Source: three-view drawing plus pictorial views. Frame: mm from the lowest corner of the part. A direction names the side the tool comes from. Give positions to 0.01 mm unless a question says otherwise; leave off trailing zeros. Order: outer loops, then holes, each group sorted by start corner. A loop starts at its lowest first (then second) coordinate and runs counter-clockwise, first axis right, second up. Notation, with made-up numbers: (7.5, 87.25) - (66.5, 87.25) arc R10 ccw to (66.5, 104.25) - close; hole circle Ø6 at (-17.75, -6.75). An arc over 180 degrees is marked (long way). Answer in a Markdown table with one row per item. Add a question column.
1. Contact query for flat-ended pins moving along their axis: pin 1 (4 mm diameter, centred on y = 3, z = 19.5, fed in from -X); pin 2 (3 mm diameter, centred on y = 7, z = 5, fed in from -X); pin 3 (2 mm diameter, centred on x = 11, z = 12, fed in from -Y). Output: stop coordinate, or through.
2. Section query A-A on x = 6.35. Return loops of the section in (y, z), and give its area (3 significant figures).
3. Access query for the marked faces 1 and 2. Directions: +Z, -Z, +X, -X, +Y, -Y. A direction counts if a zero-diameter tool reaches every point of the face in a straight line with its end or side. Return the directions, or none.
4. Ray query, line 1 (Z direction, x = 3, y = 2.75); line 2 (X direction, y = 10, z = 20.25); line 3 (X direction, y = 4, z = 12.75). Return the intervals inside material, ascending. Write a range as [from, to].
5. Section query C-C on z = 5.5. Return loops of the section in (x, y), and give its area (3 significant figures).
6. Section query D-D on y = 1. Return loops of the section in (x, z).
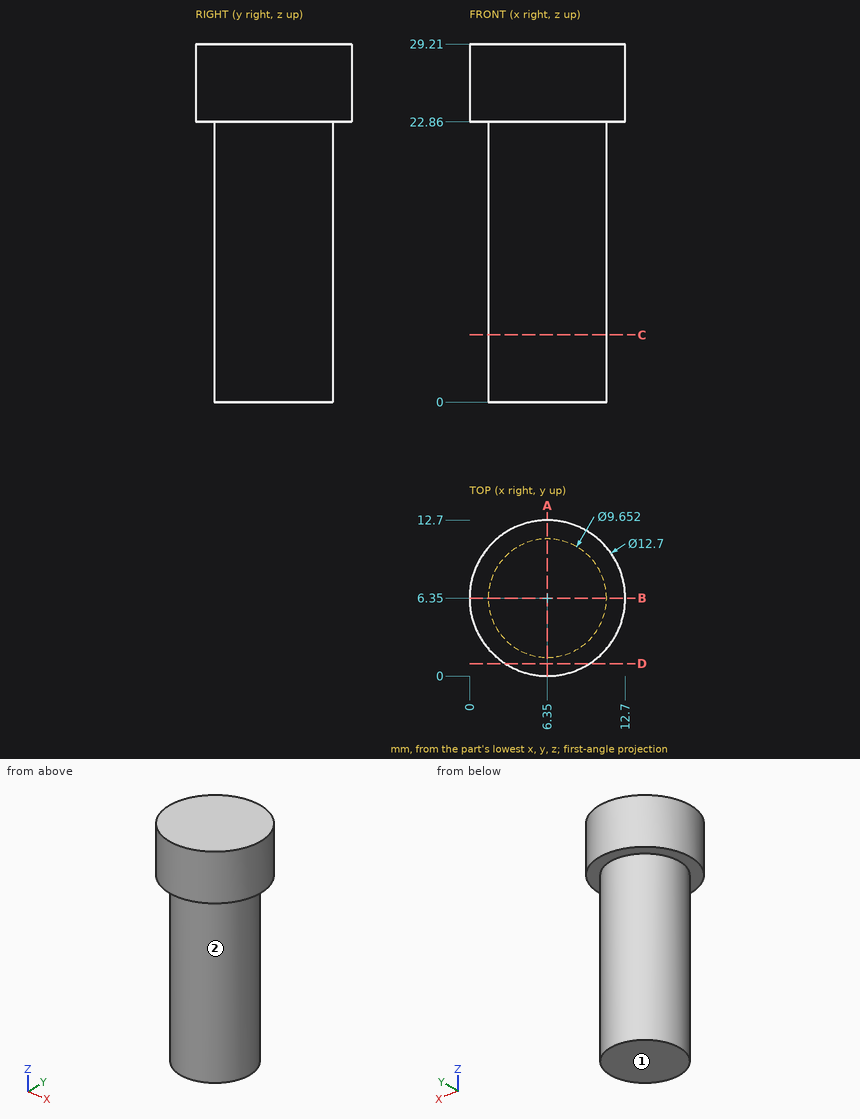
Answer:
| question | item | result |
|---|---|---|
| 1 | pin 1 | stops at x = 1.72 |
| 1 | pin 2 | stops at x = 1.52 |
| 1 | pin 3 | stops at y = 3.19 |
| 2 | outline | (0, 22.86) - (1.52, 22.86) - (1.52, 0) - (11.18, 0) - (11.18, 22.86) - (12.7, 22.86) - (12.7, 29.21) - (0, 29.21) - close |
| 2 | area | 301 mm² |
| 3 | face 1 | -Z, +X, -X, +Y, -Y |
| 3 | face 2 | -Z |
| 4 | line 1 | z = [22.86, 29.21] |
| 4 | line 2 | x = [3.19, 9.51] |
| 4 | line 3 | x = [2.13, 10.57] |
| 5 | outline | circle Ø9.65 at (6.35, 6.35) |
| 5 | area | 73.2 mm² |
| 6 | outline | (2.93, 22.86) - (9.77, 22.86) - (9.77, 29.21) - (2.93, 29.21) - close |
